Answer from the drawing. Dimensions are ordinates in mm from the lowest x, y and z of the part. A direction names the side the tool comes from. Coordinates: 2 decimals unless noted, no trailing zeros. Write each loop counter-clockwise with the first axis right and the second up, starting at its lowest first coordinate (ties: lowest second). Pieces come first, ordered by that corner, then holes.
(1) Section A-A on z = 10 is taken. Write down the section's boundary in (x, y).
(2) Section C-C on x = 14.5 is taken. Write down the section's boundary in (y, z).
(3) Find the intervals of material crossed by probe 1 along X at (y, z) = (5.75, 10); probe 2 along Y at (x, z) = (19, 4.75); probe 3 along X at (y, z) = (9.25, 11.75), in increasing order.
(4) Which of the six approach directions +Z, -Z, +X, -X, +Y, -Y give full straight-line access (tool end or side, diameter ignored) to the marked faces 1, 2 and 3?
(5) Section D-D on z = 16.5 is taken. Write down the section's boundary in (x, y).
(6) Section B-B on y = 7.25 is taken. Write down the section's boundary in (x, z), then the cut area to 3 significant figures.
(7) The mould has two halves that part along Z. Classify the marked faces 4, 5 and 6: +Z half, -Z half, draft (parallel to the pull), parting line (faces both ways), or undercut.
(8) Given pin 1 (0.5 mm diameter, centred on x = 23, y = 1, fed in from +Z); pin 2 (1.4 mm diameter, centred on x = 12.5, y = 0.5, fed in from -Z); pin 3 (5.5 mm diameter, centred on x = 19, z = 3.5, fed in from -Y), each flat-ended and moving along its own axis, determine where each tip first touches the part or whether it passes through.
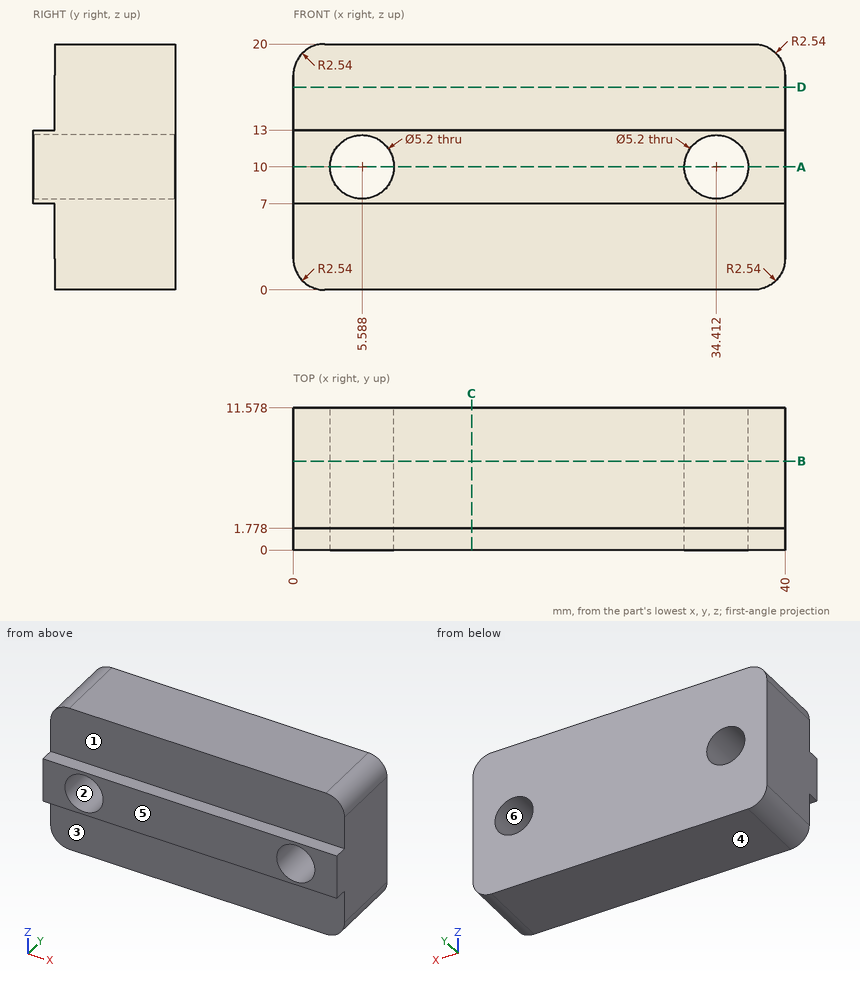
Response:
1. outline: (0, 0) - (2.99, 0) - (2.99, 11.58) - (0, 11.58) - close; (8.19, 0) - (31.81, 0) - (31.81, 11.58) - (8.19, 11.58) - close; (37.01, 0) - (40, 0) - (40, 11.58) - (37.01, 11.58) - close
2. outline: (0, 7) - (1.78, 7) - (1.78, 0) - (11.58, 0) - (11.58, 20) - (1.78, 20) - (1.78, 13) - (0, 13) - close
3. probe 1: x = 0 to 2.99, 8.19 to 31.81, 37.01 to 40
3. probe 2: y = 1.78 to 11.58
3. probe 3: x = 0 to 3.67, 7.51 to 32.49, 36.33 to 40
4. face 1: +Z, +X, -X, -Y
4. face 2: +Y, -Y
4. face 3: -Z, +X, -X, -Y
5. outline: (0, 1.78) - (40, 1.78) - (40, 11.58) - (0, 11.58) - close
6. outline: (0, 2.54) arc R2.54 ccw to (2.54, 0) - (37.46, 0) arc R2.54 ccw to (40, 2.54) - (40, 17.46) arc R2.54 ccw to (37.46, 20) - (2.54, 20) arc R2.54 ccw to (0, 17.46) - close; hole circle Ø5.2 at (5.59, 10); hole circle Ø5.2 at (34.41, 10)
6. area: 752 mm2
7. face 4: -Z half
7. face 5: draft
7. face 6: undercut
8. pin 1: stops at z = 13
8. pin 2: stops at z = 7
8. pin 3: stops at y = 1.78
